Input: part model. Units: mm. Frame: model coordinates. A direction names the side the tool comes from. Give positions to 0.01 mm unless a question says otherwise; leave off trailing zeros. Loops run counter-clockwise (first coordinate to the right, second up) from the corner with the lowest first, then second, coordinate; pieces in that order, holes last. Notation, with made-up numbers: (-31.5, 85.5) - (-21.5, 85.5) arc R25 ccw to (-21.5, 120.5) - close; hole circle Ø8 at (68, -20). An arc over 180 degrees is marked (long way). Answer as a JSON object with one key per item and string values.
from build123d import *

# Parameters (mm, degrees)
SKETCH1_R           = 2.5
BOSS_EXTRUDE1_DEPTH = 26
CUT_EXTRUDE1_START  = 2
SKETCH2_W           = 13.97289477
SKETCH2_H           = 14.193433712
CUT_EXTRUDE1_DEPTH  = 52
CHAMFER1_SIZE       = 0.5


with BuildPart() as part:
    # Sketch1 → Boss-Extrude1 (new, symmetric)
    with BuildSketch(Plane(origin=(0, 0, 0), x_dir=(1, 0, 0), z_dir=(0, 1, 0))):
        with Locations(Location((0, 0, 0), (0, 0, 90))):
            Circle(SKETCH1_R)
    extrude(amount=BOSS_EXTRUDE1_DEPTH, both=True)

    # Sketch2 → Cut-Extrude1 (cut)
    with BuildSketch(Plane(origin=(0, 0, 0), x_dir=(0, 0, -1), z_dir=(1, 0, 0)).offset(CUT_EXTRUDE1_START)):
        with Locations((0, 23.096716856)):
            Rectangle(SKETCH2_W, SKETCH2_H)
    extrude(amount=CUT_EXTRUDE1_DEPTH, mode=Mode.SUBTRACT)

    # Chamfer1
    chamfer1_edges = [part.edges().sort_by_distance(p)[0] for p in [
        (0, -26, 2.5),
        (-2.236067977, 26, 1.118033989),
        (2, 26, 0),
    ]]
    chamfer(chamfer1_edges, length=CHAMFER1_SIZE - 0.0001)  # a hair under: the kernel refuses the full size


solid = part.part
Item 1: Material intervals for line 1 (X direction, y = -2.5, z = 0.1); line 2 (X direction, y = 6, z = -2); line 3 (Z direction, x = -0.2, y = 15.5), sorted ascending. Write a range as [from, to].
Geometry check:
{"line 1": "x = [-2.5, 2.5]", "line 2": "x = [-1.5, 1.5]", "line 3": "z = [-2.49, 2.49]"}
Item 2: Mould query, pull axis Z, two halves, no side actions, for faces 3 (the face through (-2.134, 25.865, -0.075)), 4 (the face through (0, -26, 0)). Classes: released by +Z, released by -Z, zero draft, split by the parting line, or undercut.
Geometry check:
{"face 3": "split by the parting line", "face 4": "zero draft"}
Item 3: Cut plane C-C (y = 21.5). Return loops of the section in (x, z), then the cut area to 3 significant figures.
Geometry check:
{"outline": "(2, -1.5) - (2, 1.5) arc R2.5 ccw (long way) to start", "area": "18.6 mm2"}
Item 4: Contact query for a flat-ended pin moving along its axis: P1, Ø1.5, axis at y = 19.5, z = -0.5, coming from the +X side. Output: stop coordinate, or through.
Geometry check:
{"P1": "stops at x = 2"}
Item 5: Cut plane B-B (y = -12.5). Return loops of the section in (x, z), then the cut area to 3 significant figures.
Geometry check:
{"outline": "circle Ø5 at (0, 0)", "area": "19.6 mm2"}
Item 6: Cut plane A-A (z = 0). Return loops of the section in (x, y).
Geometry check:
{"outline": "(-2.5, -25.5) - (-2, -26) - (2, -26) - (2.5, -25.5) - (2.5, 16) - (2, 16) - (2, 25.5) - (1.5, 26) - (-2, 26) - (-2.5, 25.5) - close"}
Item 7: Access query for faces 1 (the face through (-2.48, 0.36, 0.33)), 2 (the face through (2, 21, 0)). Directions: +Z, -Z, +X, -X, +Y, -Y. A direction counts if a zero-diameter tool reaches every point of the face in a straight line with its end or side. Return the directions, or none.
Geometry check:
{"face 1": "+Y, -Y", "face 2": "+Z, -Z, +X, +Y"}
